Input: dimensioned drawing with shaded views. Units: mm. Origin: part minimum x, y, z. A direction names the side the tool comes from. Coordinates: 2 decimals unless noted, no trailing zeros. Order: outer loops, then holes, each group sorted by start corner. A loop starts at its lowest first (then second) coordinate and runs counter-clockwise, first axis right, second up. Notation, with made-up numbers: (64.25, -34) - (106.25, -34) arc R26 ccw to (106.25, -10) - close; hole circle Ø10 at (20.5, 19). An arc over 180 degrees is marked (long way). Answer as CSV lines item,"result". Start each with the question number.
Item 1: Section C-C (z = 22). Output: boundary loops of the cut face in (x, y), and give its area (4 significant figures).
Item 2: Section B-B (x = 16.5). Output: boundary loops of the cut face in (y, z), and give its area (3 significant figures).
Item 3: Section A-A (y = 6.5). Output: boundary loops of the cut face in (x, z).
Item 4: Material intervals for line 1 along Z through (x, y) = (39, 18); line 2 along Y through (x, z) = (47, 23); line 3 along X through (y, z) = (13.5, 14.5), sorted ascending.
Item 5: First-contact query: pin 1 (12 mm diameter, centred on x = 40, y = 12.5, fed in from +Z); pin 2 (1.5 mm diameter, centred on y = 14.5, z = 19.5, fed in from -X); pin 3 (4.5 mm diameter, centred on x = 25.92, y = 5.21, fed in from -Z). Flat tips, straight axial feed; report the tip coordinate or a pass-through.
Item 6: Access query for the marked faces 1, 2 and 3. Directions: +Z, -Z, +X, -X, +Y, -Y. A direction counts if a zero-diameter tool reaches every point of the face in a straight line with its end or side. Return the directions, or none.
Item 7: Section D-D (y = 19.5). Output: boundary loops of the cut face in (x, z).
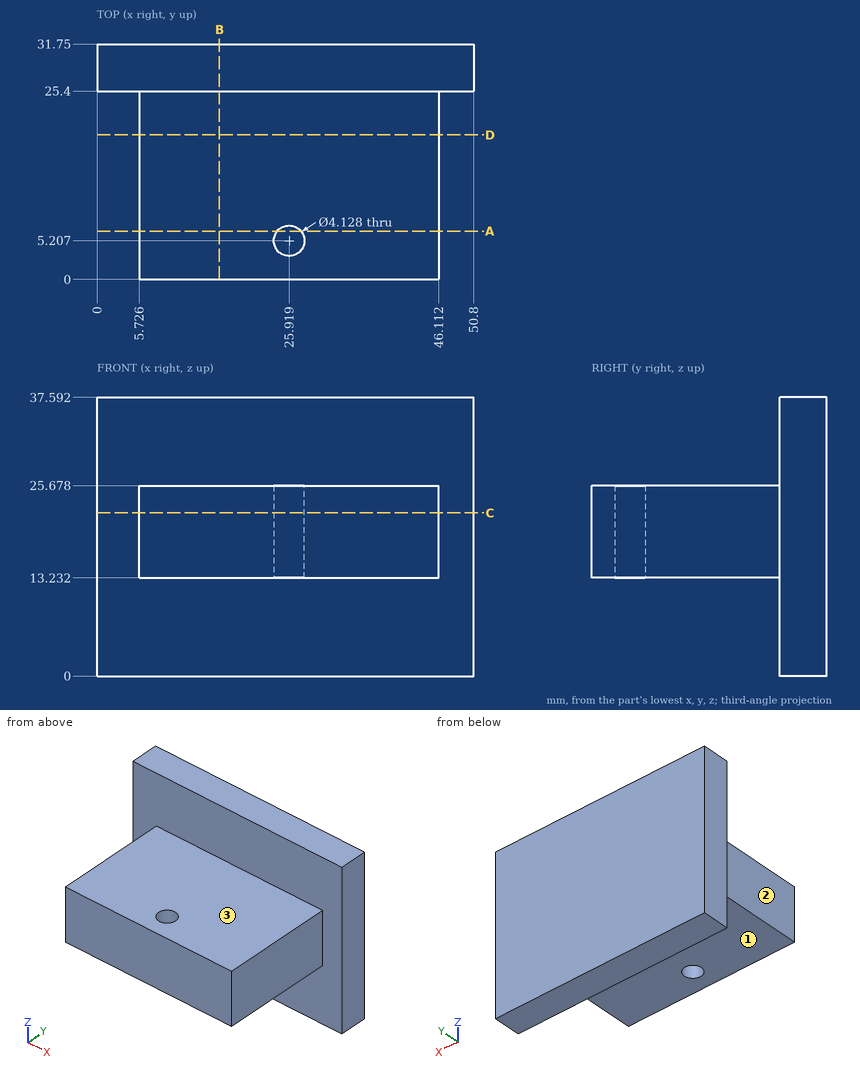
Determined:
1,outline,"(0, 25.4) - (5.73, 25.4) - (5.73, 0) - (46.11, 0) - (46.11, 25.4) - (50.8, 25.4) - (50.8, 31.75) - (0, 31.75) - close; hole circle Ø4.13 at (25.92, 5.21)"
1,area,"1,335 mm^2"
2,outline,"(0, 13.23) - (25.4, 13.23) - (25.4, 0) - (31.75, 0) - (31.75, 37.59) - (25.4, 37.59) - (25.4, 25.68) - (0, 25.68) - close"
2,area,"555 mm^2"
3,outline,"(5.73, 13.23) - (24.31, 13.23) - (24.31, 25.68) - (5.73, 25.68) - close; (27.53, 13.23) - (46.11, 13.23) - (46.11, 25.68) - (27.53, 25.68) - close"
4,line 1,"z = 13.23 to 25.68"
4,line 2,"y = 25.4 to 31.75"
4,line 3,"x = 5.73 to 46.11"
5,pin 1,"stops at z = 25.68"
5,pin 2,"stops at x = 5.73"
5,pin 3,"stops at z = 13.23"
6,face 1,"-Z, +X, -X, -Y"
6,face 2,"+Z, -Z, -X, -Y"
6,face 3,"+Z, +X, -X, -Y"
7,outline,"(5.73, 13.23) - (46.11, 13.23) - (46.11, 25.68) - (5.73, 25.68) - close"
